Read the model definition and answer for the solid it produces. Units are mm, in the model's axes. A direction names the side the tool comes from. Coordinates: 2 decimals unless noted, no trailing zeros. Write each loop counter-clockwise with the first axis right and the second up, starting at its lowest first coordinate (ties: lowest second). Pieces come first, ordered by that corner, then holes.
(1) Given pin 1 (2 mm diameter, centred on x = 26, y = -12, fed in from +Z); pin 2 (1 mm diameter, centred on x = 14.5, y = -7.5, fed in from +Z); pin 3 (3 mm diameter, centred on x = 23.5, z = 4, fed in from -Y), each flat-ended and moving along its own axis, determine where each tip first touches the part or whether it passes through.
(2) Section A-A on y = -32.5 is taken. Write down the section's boundary in (x, z), then the cut area to 3 significant figures.
(3) Section B-B on z = 3.5 is taken. Write down the section's boundary in (x, y), then the cut area to 3 significant figures.
(4) Find the intervals of material crossed by probe 1 along X at (y, z) = (-36, 7.25); probe 2 along Y at (x, z) = (30.5, 3); probe 3 along Y at (x, z) = (33.5, 19), in increasing order.
(5) The mould has two halves that part along X. Classify faces 1 (the flat face through (19, -19, 0)), 2 (the flat face through (38.1, -14, 7)), 3 (the flat face through (19, -31.75, 5)): +X half, -X half, draft (parallel to the pull), parting line (faces both ways), or undercut.
(6) Section D-D on x = 35 is taken. Write down the section's boundary in (y, z).
(7) Section C-C on y = -47 is taken. Write down the section's boundary in (x, z).
(8) Which of the six approach directions +Z, -Z, +X, -X, +Y, -Y give full straight-line access (tool end or side, diameter ignored) to faces 4 (the flat face through (6.35, -37, 3)), 5 (the flat face through (19, 0, 13))?
from build123d import *

# Parameters (mm, degrees)
F1_DEPTH = 25.4
F3_DEPTH = 38.101


with BuildPart() as f1:
    # F0 (on Top) → F1 (new body)
    with BuildSketch(Plane.XY):
        Polygon((38.1, 0), (0, 0), (0, -50.8), (6.35, -50.8), (6.35, -31.75), (31.75, -31.75), (31.75, -50.8), (38.1, -50.8), align=None)
    extrude(amount=F1_DEPTH)

    # F2 (on face) → F3 (cut, through all)
    with BuildSketch(Plane.YZ.offset(38.1)):
        Polygon((-50.8, 25.4), (-50.8, 0), (0, 25.4), align=None)
    extrude(amount=-F3_DEPTH, mode=Mode.SUBTRACT)


solid = f1.part
Response:
1. pin 1: stops at z = 19.9
1. pin 2: stops at z = 21.9
1. pin 3: stops at y = -31.75
2. outline: (0, 0) - (6.35, 0) - (6.35, 9.15) - (0, 9.15) - close; (31.75, 0) - (38.1, 0) - (38.1, 9.15) - (31.75, 9.15) - close
2. area: 116 mm2
3. outline: (0, -43.8) - (6.35, -43.8) - (6.35, -31.75) - (31.75, -31.75) - (31.75, -43.8) - (38.1, -43.8) - (38.1, 0) - (0, 0) - close
3. area: 1,360 mm2
4. probe 1: x = 0 to 6.35, 31.75 to 38.1
4. probe 2: y = -31.75 to 0
4. probe 3: y = -12.8 to 0
5. face 1: draft
5. face 2: +X half
5. face 3: undercut
6. outline: (-50.8, 0) - (0, 0) - (0, 25.4) - close
7. outline: (0, 0) - (6.35, 0) - (6.35, 1.9) - (0, 1.9) - close; (31.75, 0) - (38.1, 0) - (38.1, 1.9) - (31.75, 1.9) - close
8. face 4: +Z, -Z, -Y
8. face 5: +Z, -Z, +X, -X, +Y
